Check sheet for the modelled part. Datum: model origin and axes. Units: mm. Round coordinates to 2 decimals unless told otherwise and drop trailing zeros. Write each loop counter-clockwise with the first axis right and the second up, starting at its lowest first coordinate (ties: lowest second). Pieces come first, ordered by that corner, then holes.
Item 1: Go/stop test with flat-tipped pins: pin 1 Ø2.5 at (x, z) = (0, -9.5) entering from -Y; pin 2 Ø3.5 at (x, z) = (0, 17) entering from +Y; pin 3 Ø1 at (x, y) = (10, 1) entering from -Z; pin 4 Ø1 at (y, z) = (1.5, -3) entering from -X. Record where each tip stops, or that it passes through.
Item 2: Cross-section at D-D on z = 14. Enter the section's corners in (x, y) (3 decimals), plus the area to 3 significant figures.
Item 3: Cross-section at B-B on y = 0.45. Count the separate pieces of the cut face and the enclosed holes in it, plus the area to 3 significant figures.
Item 4: Material ranges on line 1 (Z direction, x = -8, y = 0.35); line 2 (Z direction, x = -12, y = 1.1), recorded low to high.
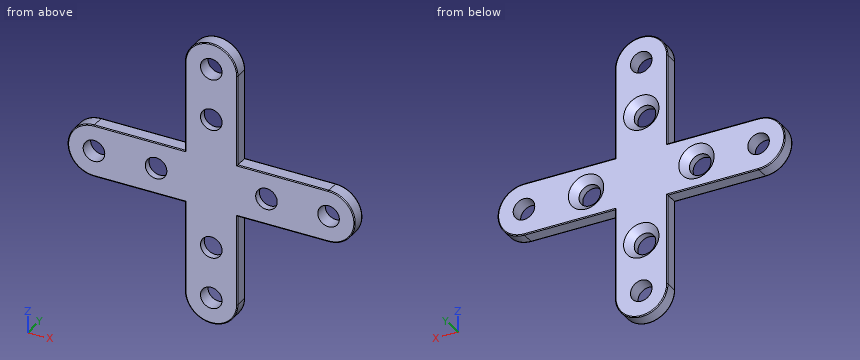
from build123d import *

# Parameters (mm, degrees)
SKETCH1_R           = 1.5625
BOSS_EXTRUDE1_DEPTH = 2
CIRPATTERN1_COUNT   = 2
CIRPATTERN1_ANGLE   = 90
SKETCH2_R           = 1.5625
CUT_EXTRUDE1_DEPTH  = 2
CHAMFER1_SIZE       = 1
FILLET1_R           = 0.125


with BuildPart() as part:
    # Sketch1 → Boss-Extrude1 (new body)
    with BuildSketch(Plane(origin=(0, 0, 0), x_dir=(1, 0, 0), z_dir=(0, 1, 0))):
        with BuildLine():
            Line((-3.8, -17), (-3.8, 17))
            ThreePointArc((-3.8, 17), (0, 20.8), (3.8, 17))
            Line((3.8, 17), (3.8, -17))
            ThreePointArc((3.8, -17), (0, -20.8), (-3.8, -17))
        make_face()
        with Locations(Location((0, 17, 0), (0, 0, 270))):
            Circle(SKETCH1_R, mode=Mode.SUBTRACT)
        with Locations(Location((0, -17, 0), (0, 0, 90))):
            Circle(SKETCH1_R, mode=Mode.SUBTRACT)
    boss_extrude1 = extrude(amount=BOSS_EXTRUDE1_DEPTH)

    # CirPattern1: Boss-Extrude1 ×2 about axis
    cirpattern1_axis = Axis((0, 0, 0), (0, 1, 0))
    for i in range(1, CIRPATTERN1_COUNT):
        add(boss_extrude1.rotate(cirpattern1_axis, i * CIRPATTERN1_ANGLE / (CIRPATTERN1_COUNT - 1)))

    # Sketch2 → Cut-Extrude1 (cut)
    with BuildSketch(Plane(origin=(0, 0, 0), x_dir=(1, 0, 0), z_dir=(0, 1, 0))):
        with Locations(Location((0, 9.5, 0), (0, 0, 270))):
            Circle(SKETCH2_R)
        with Locations(Location((8, 0, 0), (0, 0, 270))):
            Circle(SKETCH2_R)
        with Locations(Location((0, -9.5, 0), (0, 0, 90))):
            Circle(SKETCH2_R)
        with Locations(Location((-8, 0, 0), (0, 0, 90))):
            Circle(SKETCH2_R)
    extrude(amount=CUT_EXTRUDE1_DEPTH, mode=Mode.SUBTRACT)

    # Chamfer1
    chamfer1_edges = [part.edges().sort_by_distance(p)[0] for p in [
        (0, 2, -11.0625),
        (8, 2, -1.5625),
        (0, 2, 11.0625),
        (-8, 2, 1.5625),
    ]]
    chamfer(chamfer1_edges, length=CHAMFER1_SIZE)

    # Fillet1
    fillet1_edges = [part.edges().sort_by_distance(p)[0] for p in [
        (0, 2, -20.8),
        (-3.8, 2, -10.4),
        (-3.8, 0, 10.4),
        (-3.8, 2, 10.4),
        (3.8, 0, -10.4),
        (3.8, 2, -10.4),
        (10.4, 2, 3.8),
        (20.8, 2, 0),
        (10.4, 2, -3.8),
        (-10.4, 2, -3.8),
        (-20.8, 2, 0),
        (-10.4, 2, 3.8),
        (10.4, 0, -3.8),
        (-10.4, 0, -3.8),
        (10.4, 0, 3.8),
        (-10.4, 0, 3.8),
        (20.8, 0, 0),
        (-20.8, 0, 0),
        (0, 2, 20.8),
        (-3.8, 0, -10.4),
        (0, 0, -20.8),
        (3.8, 0, 10.4),
        (0, 0, 20.8),
        (3.8, 2, 10.4),
    ]]
    fillet(fillet1_edges, radius=FILLET1_R)


solid = part.part
Response values:
1. pin 1: passes through
1. pin 2: stops at y = 2
1. pin 3: stops at z = -3.8
1. pin 4: stops at x = -19.86
2. outline: (-3.8, 0.125) arc R0.125 ccw to (-3.675, 0) - (3.675, 0) arc R0.125 ccw to (3.8, 0.125) - (3.8, 1.875) arc R0.125 ccw to (3.675, 2) - (-3.675, 2) arc R0.125 ccw to (-3.8, 1.875) - close
2. area: 15.2 mm2
3. separate pieces: 1
3. enclosed holes: 8
3. area: 488 mm2
4. line 1: z = -3.8 to -1.56, 1.56 to 3.8
4. line 2: z = -3.8 to 3.8
